Design review of the part shown in the three views and the two pictorial views. Dimensions are in mm from the part's minimum x, y and z. Coordinates: 2 decimals unless noted, no trailing zeros. Loops run counter-clockwise (first coordinate to the right, second up) from the corner with the lowest first, then second, coordinate; pieces in that order, holes last. Notation, with made-up numbers: M 6,63 L 36,63 A9 cw 36,73 Z; hole C 24.5,3.25 d2. An arc over 180 degrees is marked long. Use one line per item in the form item = value.
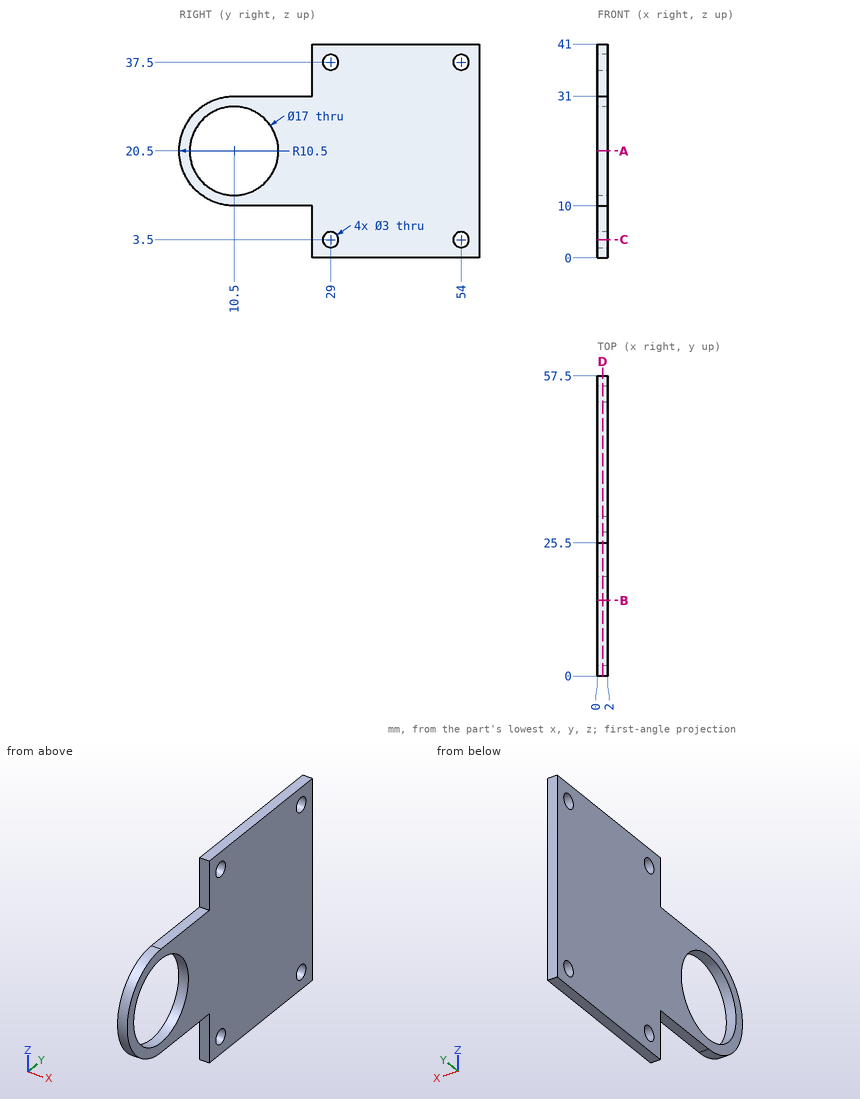
1. Insertion check: P1, Ø1, axis at x = 1, y = 21, coming from the -Z side; P2, Ø1, axis at x = 0.5, z = 6.5, coming from the -Y side. Each pin has a flat end and moves straight along its axis. Give the tip position at first contact, or say it passes through.
Response values:
P1 = 10
P2 = 25.5
2. Add section B-B (y = 14.5). State the section outline as (x, z) points.
Response values:
outline = M 0,10 L 2,10 L 2,13 L 0,13 Z; M 0,28 L 2,28 L 2,31 L 0,31 Z
3. Add section D-D (x = 1). State the section outline as (y, z) points.
Response values:
outline = M 10.5,10 L 25.5,10 L 25.5,0 L 57.5,0 L 57.5,41 L 25.5,41 L 25.5,31 L 10.5,31 A10.5 ccw Z; hole C 10.5,20.5 d17; hole C 29,3.5 d3; hole C 29,37.5 d3; hole C 54,3.5 d3; hole C 54,37.5 d3
4. Wall thickness on line 1 along Y through (x, z) = (1.4, 37.5); line 2 along Y through (x, z) = (1.05, 20.5); line 3 along Z through (x, y) = (0.2, 10): over which ranges is each line inside the solid? List them lowest first. Write a range as from..to.
Response values:
line_1 = 25.5..27.5, 30.5..52.5, 55.5..57.5
line_2 = 0..2, 19..57.5
line_3 = 10.01..12.01, 28.99..30.99
5. Add section C-C (z = 3.5). State the section outline as (x, y) points, then the cut area to 3 significant figures.
Response values:
outline = M 0,25.5 L 2,25.5 L 2,27.5 L 0,27.5 Z; M 0,30.5 L 2,30.5 L 2,52.5 L 0,52.5 Z; M 0,55.5 L 2,55.5 L 2,57.5 L 0,57.5 Z
area = 52.0 mm^2
6. Add section A-A (z = 20.5). State the section outline as (x, y) points.
Response values:
outline = M 0,0 L 2,0 L 2,2 L 0,2 Z; M 0,19 L 2,19 L 2,57.5 L 0,57.5 Z
